from build123d import *

# Parameters (mm, degrees)
BLOCK_START            = 465
BLOCK_1_DEPTH          = 30
BLOCK_EDGE_FILLET_1_R  = 7
EXTRUDE_START          = -17
EXTRUDE_SKETCH_1_R     = 7
EXTRUDE_1_DEPTH        = 34
EXTRUDE_ROTATE_1_ANGLE = 90
EXTRUDE_SKETCH_2_R     = 7
EXTRUDE_2_DEPTH        = 34
EXTRUDE_ROTATE_2_ANGLE = 90


with BuildPart() as part:
    # Block sketch 1 → Block 1 (new body)
    with BuildSketch(Plane.XY.offset(BLOCK_START)):
        with BuildLine():
            Line((358, -132), (632, -132))
            ThreePointArc((632, -132), (642.606601718, -127.606601718), (647, -117))
            Line((647, -117), (647, 117))
            ThreePointArc((647, 117), (642.606601718, 127.606601718), (632, 132))
            Line((632, 132), (358, 132))
            ThreePointArc((358, 132), (347.393398282, 127.606601718), (343, 117))
            Line((343, 117), (343, -117))
            ThreePointArc((343, -117), (347.393398282, -127.606601718), (358, -132))
        make_face()
    extrude(amount=BLOCK_1_DEPTH)

    # Block edge fillet 1
    block_edge_fillet_1_edges = [part.edges().sort_by_distance(p)[0] for p in [
        (647, 0, 465),
        (642.606601718, -127.606601718, 465),
        (495, -132, 465),
        (347.393398282, -127.606601718, 465),
        (642.606601718, -127.606601718, 495),
        (647, 0, 495),
        (642.606601718, 127.606601718, 495),
        (495, 132, 495),
        (347.393398282, 127.606601718, 495),
        (343, 0, 495),
        (347.393398282, -127.606601718, 495),
        (343, 0, 465),
        (495, -132, 495),
        (347.393398282, 127.606601718, 465),
        (495, 132, 465),
        (642.606601718, 127.606601718, 465),
    ]]
    fillet(block_edge_fillet_1_edges, radius=BLOCK_EDGE_FILLET_1_R)


with BuildPart() as body_2:
    # Extrude sketch 1 → Extrude 1 (new body)
    with BuildSketch(Plane.XY.offset(EXTRUDE_START)):
        Circle(EXTRUDE_SKETCH_1_R)
    extrude(amount=EXTRUDE_1_DEPTH)


with BuildPart() as body_2_1:
    # Extrude rotate 1: moved
    add(body_2.part.rotate(Axis((0, 0, 0), (0, 1, 0)), EXTRUDE_ROTATE_1_ANGLE))


with BuildPart() as body_2_2:
    # Extrude place 1: moved
    add(body_2_1.part.moved(Location((415, 136, 467))))


with BuildPart() as body_3:
    # Extrude sketch 2 → Extrude 2 (new body)
    with BuildSketch(Plane.XY.offset(EXTRUDE_START)):
        Circle(EXTRUDE_SKETCH_2_R)
    extrude(amount=EXTRUDE_2_DEPTH)


with BuildPart() as body_3_1:
    # Extrude rotate 2: moved
    add(body_3.part.rotate(Axis((0, 0, 0), (0, 1, 0)), EXTRUDE_ROTATE_2_ANGLE))


with BuildPart() as body_3_2:
    # Extrude place 2: moved
    add(body_3_1.part.moved(Location((575, 136, 467))))


with BuildPart() as part_1:
    add(part.part)

    # Combine (weld / assembly of features): union body 3, body 2
    add(body_3_2.part)
    add(body_2_2.part)


solid = part_1.part
Design review of the part built by this model. Coordinates are the model's own, in mm. A direction names the side the tool comes from. Round coordinates to 2 decimals unless told otherwise and drop trailing zeros. Order: outer loops, then holes, each group sorted by start corner. A loop starts at its lowest first (then second) coordinate and runs counter-clockwise, first axis right, second up. Notation, with made-up numbers: M 22,-9.75 L 70,-9.75 A19 ccw 70,20.25 Z; hole C 19,55.5 d9. An arc over 180 degrees is marked long. Answer as CSV lines item,"result". Start each with the question number.
1) Add section C-C (y = -26). Give the boundary of the cut face in (x, z).
2) For pin 1 Ø15.5 at (y, z) = (134, 464) entering from -X; pin 2 Ø7 at (y, z) = (137.5, 465) entering from -X; pin 3 Ø17.5 at (x, z) = (452, 478) entering from +Y, all flat-tipped, find the tip position at first contact; note any pin that passes through.
3) Add section B-B (x = 526.5). Give the boundary of the cut face in (y, z).
4) Wall thickness on line 1 along Y through (x, z) = (554, 481.5); line 2 along Z through (x, y) = (579, 88); line 3 along X through (y, z) = (-70, 469.5): over which ranges is each line inside the solid? List them lowest first. Write a range as [from, to].
5) Add section A-A (y = 136). Give the boundary of the cut face in (x, z), then the cut area to 3 significant figures.
6) Add section D-D (x = 586). Give the boundary of the cut face in (y, z).
7) Tool access review of faces 1 (the face through (493, 2, 465)), 2 (the face through (345, -1.6, 467.1)): name each direction out of +Z, -Z, +X, -X, +Y, -Y from which nothing blocks a thin tool from reaching the whole face with its end or side.
Resolved:
1,outline,"M 343,472 A7 ccw 350,465 L 640,465 A7 ccw 647,472 L 647,488 A7 ccw 640,495 L 350,495 A7 ccw 343,488 Z"
2,pin 1,"x = 348.86"
2,pin 2,"x = 398"
2,pin 3,"y = 132"
3,outline,"M -132,472 A7 ccw -125,465 L 125,465 A7 ccw 132,472 L 132,488 A7 ccw 125,495 L -125,495 A7 ccw -132,488 Z"
4,line 1,"[-132, 132]"
4,line 2,"[465, 495]"
4,line 3,"[343.46, 646.54]"
5,outline,"M 398,460 L 432,460 L 432,474 L 398,474 Z; M 558,460 L 592,460 L 592,474 L 558,474 Z"
5,area,"952 mm^2"
6,outline,"M -132,472 A7 ccw -125,465 L 125,465 A7 ccw 129.04,466.28 A7 ccw long 132,472.74 L 132,488 A7 ccw 125,495 L -125,495 A7 ccw -132,488 Z"
7,face 1,"-Z, +X, -X, -Y"
7,face 2,"-Z, -X, +Y, -Y"
